Source: CAD feature listing. Evaluate the final solid. Frame: model axes, mm. Face numbers are marked on the shaded views. A direction names the side the tool comes from. Give positions to 0.01 mm unless a question says otherwise; leave off trailing zeros. Loops run counter-clockwise (first coordinate to the right, second up) from the corner with the lowest first, then second, coordinate; pieces in that order, holes last. Notation, with made-up numbers: M 52.5,84 L 101.5,84 A12 cw 101.5,102 Z; hole C 58,39 d7. An arc over 180 degrees is marked long. Write item = value, one per line.
Autodesk Inventor part; units mm, degrees
ref_plane "YZ Plane" through (0, 0, 0) normal (1, 0, 0) x (0, 1, 0)
ref_plane "XZ Plane" through (0, 0, 0) normal (0, 1, 0) x (-1, 0, 0)
ref_plane "XY Plane" through (0, 0, 0) normal (0, 0, 1) x (1, 0, 0)
sketch "Sketch1" plane through (0, 0, 0) normal (1, 0, 0) x (0, 1, 0)
  circle A0 centre (0, 0) radius 2.75
  line L0 (-2.75, 0) -> (2.15, 0)
  line L1 (2.15, 0) -> (2.15, -1.7146)
  line L2 (2.15, 0) -> (2.15, 1.7146)
  circle A1 centre (0, 0) radius 5.25
  line L3 (15, 1.5) -> (-15, 1.5)
  line L4 (-15, 1.5) -> (-15, -1.5)
  line L5 (-15, -1.5) -> (15, -1.5)
  line L6 (15, -1.5) -> (15, 1.5)
  line L7 (15, 1.5) -> (-15, -1.5) construction
  line L8 (-15, 1.5) -> (15, -1.5) construction
  point P0 (5.0312, 1.5)
  point P1 (-5.0312, 1.5)
  point P2 (-5.0312, -1.5)
  point P3 (5.0312, -1.5)
  dimension "d0" = 5.5
  dimension "d3" = 4.9
  dimension "d4" = 2.5
  dimension "d5" = 30
  dimension "d6" = 3
extrude "Extrusion1" add sketch "Sketch1" along normal blind 5 contours A0 L5 L1 L2 L3 | A0 L3 A1 L5 | L3 L2 A0 | A0 L3 A1 | L5 A1 A0 | A0 L1 L5 | L3 L6 L5 A1 | A0 L5 A1 L3 | A1 L5 L4 L3 picked at (2.168, 1.6198) picked at (2.168, -1.6198)
properties part number "dshaft_fit_test"
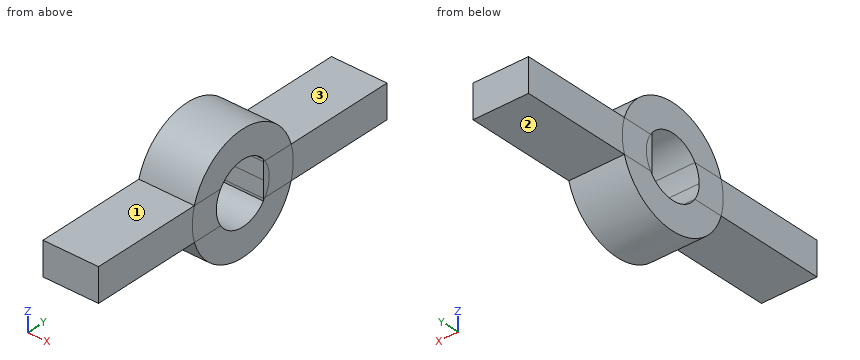
1. First-contact query: pin 1 Ø3 at (x, y) = (0.5, 6) entering from -Z; pin 2 Ø2.5 at (x, y) = (2, 9) entering from -Z; pin 3 Ø2.5 at (x, y) = (2, 12) entering from +Z. Flat tips, straight axial feed; report the tip coordinate or a pass-through.
Derived:
pin_1 = -2.7
pin_2 = -1.5
pin_3 = 1.5
2. Cut plane A-A, the plane x = 1.15. Return the cut outline in (y, z).
Derived:
outline = M -15,-1.5 L -5.03,-1.5 A5.25 ccw 5.03,-1.5 L 15,-1.5 L 15,1.5 L 5.03,1.5 A5.25 ccw -5.03,1.5 L -15,1.5 Z; hole M 2.15,-1.71 L 2.15,1.71 A2.75 ccw long Z
3. Cut plane C-C, the plane y = 1.25. Return the cut outline in (x, z), then the cut area to 3 significant figures.
Derived:
outline = M 0,-5.1 L 5,-5.1 L 5,-2.45 L 0,-2.45 Z; M 0,2.45 L 5,2.45 L 5,5.1 L 0,5.1 Z
area = 26.5 mm²
4. Cut plane D-D, the plane y = 6.75. Return the cut outline in (x, z).
Derived:
outline = M 0,-1.5 L 5,-1.5 L 5,1.5 L 0,1.5 Z
5. Material intervals for probe 1 along Z at (x, y) = (1.6, -12.5); probe 2 along Y at (x, z) = (4.4, 0.75); probe 3 along Z at (x, y) = (3.95, -0.5), sorted ascending. Write a range as from..to.
Derived:
probe_1 = -1.5..1.5
probe_2 = -15..-2.65, 2.15..15
probe_3 = -5.23..-2.7, 2.7..5.23
6. Cut plane B-B, the plane z = -1. Return the cut outline in (x, y).
Derived:
outline = M 0,-15 L 5,-15 L 5,-2.56 L 0,-2.56 Z; M 0,2.15 L 5,2.15 L 5,15 L 0,15 Z
7. Reachability of the marked faces 1, 2 and 3 from +Z, -Z, +X, -X, +Y, -Y: full face, straight path, thin tool, end or side. Return the list, or none.
Derived:
face_1 = +Z, +X, -X, -Y
face_2 = -Z, +X, -X, +Y
face_3 = +Z, +X, -X, +Y
